Could you check a few things on this drawing? It's one solid part, dimensions in mm from its lowest x, y, z. A direction names the side the tool comes from. Give positions to 0.01 mm unless a question says otherwise; leave off trailing zeros. Order: outer loops, then holes, each group sorted by start corner. A loop starts at its lowest first (then second) coordinate and runs counter-clockwise, first axis right, second up. Notation, with made-up numbers: (80.5, 73) - (101.5, 73) arc R26 cw to (101.5, 104) - close; hole circle Ø6 at (45, 72). An arc over 180 degrees is marked (long way). Put each result on its own line as item: value.
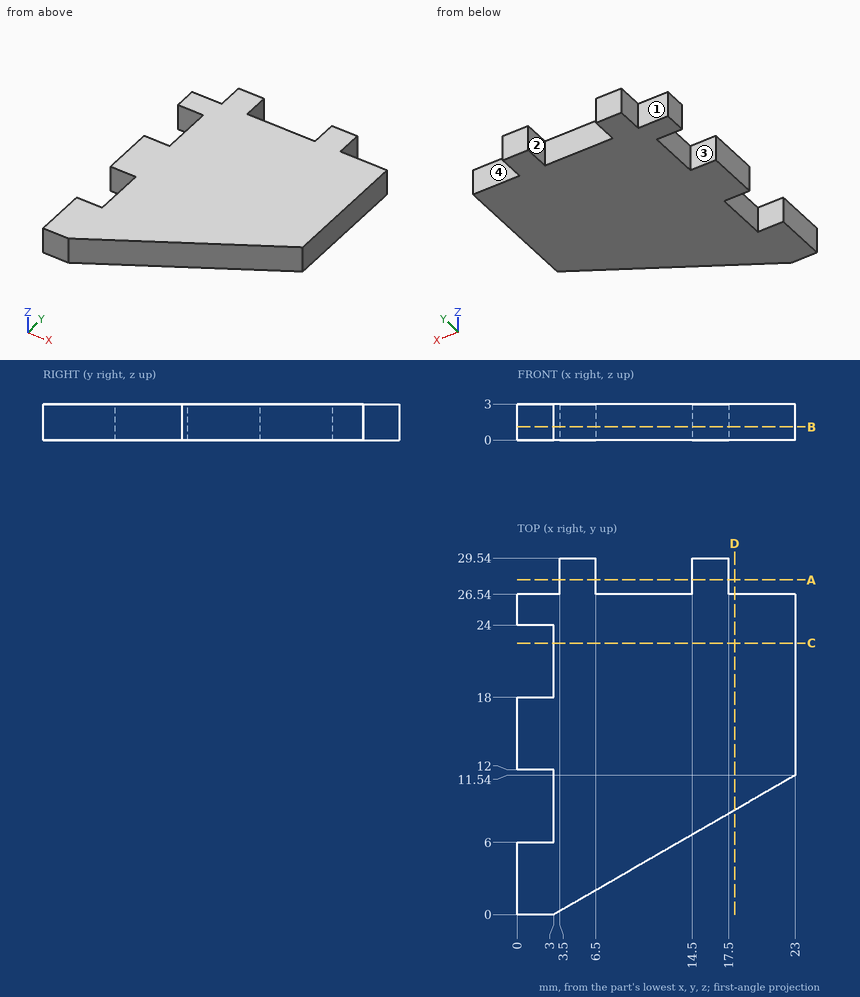
1) Suppose I cut it at B-B, the plane z = 1.1. List the corners of the cut face in (x, y) for me.
Filled in:
outline: (0, 0) - (3, 0) - (23, 11.54) - (23, 26.54) - (17.5, 26.54) - (17.5, 29.54) - (14.5, 29.54) - (14.5, 26.54) - (6.5, 26.54) - (6.5, 29.54) - (3.5, 29.54) - (3.5, 26.54) - (0, 26.54) - (0, 24) - (3, 24) - (3, 18) - (0, 18) - (0, 12) - (3, 12) - (3, 6) - (0, 6) - close
2) If I drill on line 1 (X direction, y = 19.5, z = 1.7); line 2 (X direction, y = 2, z = 2.85); line 3 (Y direction, x = 9, z = 0.85), over which ranges is the centre line in solid material (lowest first)? Write a range as [from, to].
Filled in:
line 1: x = [3, 23]
line 2: x = [0, 6.47]
line 3: y = [3.46, 26.54]
3) Suppose I cut it at A-A, the plane y = 27.75. List the corners of the cut face in (x, z) for me.
Filled in:
outline: (3.5, 0) - (6.5, 0) - (6.5, 3) - (3.5, 3) - close; (14.5, 0) - (17.5, 0) - (17.5, 3) - (14.5, 3) - close
4) I'm going to push flat-ended pins straight in: pin 1 (0.9 mm diameter, centred on y = 27.5, z = 1, fed in from +X); pin 2 (1.5 mm diameter, centred on x = 1.5, z = 2, fed in from -Y); pin 3 (0.9 mm diameter, centred on x = 2.5, z = 1.5, fed in from +Y); pin 4 (1.5 mm diameter, centred on y = 27.5, z = 2, fed in from -X). Where does each tip first touch, or does it pass through?
Filled in:
pin 1: stops at x = 17.5
pin 2: stops at y = 0
pin 3: stops at y = 26.54
pin 4: stops at x = 3.5
5) Suppose I cut it at C-C, the plane y = 22.5. List the corners of the cut face in (x, z) for me.
Filled in:
outline: (3, 0) - (23, 0) - (23, 3) - (3, 3) - close
6) Suppose I cut it at D-D, the plane x = 18. List the corners of the cut face in (y, z) for me (3 decimals), and give its area (3 significant figures).
Filled in:
outline: (8.655, 0) - (26.54, 0) - (26.54, 3) - (8.655, 3) - close
area: 53.7 mm^2
7) Which directions (+Z, -Z, +X, -X, +Y, -Y) give clear straight access to the entire face, cutting with the end or side of a thin tool? Please do the marked faces 1, 2, 3 and 4.
Filled in:
face 1: +Z, -Z, -X, +Y
face 2: +Z, -Z, +Y
face 3: +Z, -Z, -X
face 4: +Z, -Z, +X, +Y
